```python
from build123d import *

# Parameters (mm, degrees)
SKETCH1_W           = 100
SKETCH1_H           = 100
BOSS_EXTRUDE1_DEPTH = 1.6
CUT_EXTRUDE1_DEPTH  = 1.6
SKETCH7_R           = 1.5875
CUT_EXTRUDE2_DEPTH  = 1.6
SKETCH8_W           = 32
SKETCH8_H           = 6
BOSS_EXTRUDE2_DEPTH = 5
BOSS_EXTRUDE3_DEPTH = 2
SKETCH12_W          = 20
SKETCH12_H          = 6
BOSS_EXTRUDE5_DEPTH = 2


with BuildPart() as part:
    # Sketch1 → Boss-Extrude1 (new body)
    with BuildSketch(Plane.XY):
        with Locations((15.275668243, 27.330907947)):
            Rectangle(SKETCH1_W, SKETCH1_H)
    extrude(amount=BOSS_EXTRUDE1_DEPTH)

    # Sketch2 → Cut-Extrude1 (cut)
    with BuildSketch(Plane.XY.offset(1.6)):
        Polygon((-34.724331757, 57.330907947), (-14.724331757, 77.330907947), (-34.724331757, 77.330907947), align=None)
        Polygon((-34.724331757, -2.669092053), (-14.724331757, -22.669092053), (-34.724331757, -22.669092053), align=None)
        Polygon((45.275668243, 77.330907947), (65.275668243, 57.330907947), (65.275668243, 77.330907947), align=None)
        Polygon((65.275668243, -2.669092053), (45.275668243, -22.669092053), (65.275668243, -22.669092053), align=None)
    extrude(amount=-CUT_EXTRUDE1_DEPTH, mode=Mode.SUBTRACT)

    # Sketch7 → Cut-Extrude2 (cut)
    with BuildSketch(Plane.XY.offset(1.6)):
        with Locations((-25.724331757, 34.330907947)):
            Circle(SKETCH7_R)
        with Locations((-16.624331757, 64.904907947)):
            Circle(SKETCH7_R)
        with Locations((34.275668243, 69.330907947)):
            Circle(SKETCH7_R)
        with Locations((54.275668243, 29.330907947)):
            Circle(SKETCH7_R)
        with Locations((62.999668243, 19.180907947)):
            Circle(SKETCH7_R)
        with Locations((-4.300331757, -20.219092053)):
            Circle(SKETCH7_R)
        with Locations((4.275668243, -5.669092053)):
            Circle(SKETCH7_R)
    extrude(amount=-CUT_EXTRUDE2_DEPTH, mode=Mode.SUBTRACT)

    # Sketch8 → Boss-Extrude2 (add)
    with BuildSketch(Plane.XY.offset(1.6)):
        with Locations((12.949668243, 27.580907947)):
            Rectangle(SKETCH8_W, SKETCH8_H)
    extrude(amount=BOSS_EXTRUDE2_DEPTH)

    # Sketch10 → Boss-Extrude3 (add)
    with BuildSketch(Plane.XY.offset(1.6)):
        Polygon((-34.724331757, 57.330907947), (-14.724331757, 77.330907947), (-12.603011413, 75.209587604), (-32.603011413, 55.209587604), align=None)
        Polygon((45.275668243, 77.330907947), (65.275668243, 57.330907947), (63.154347899, 55.209587604), (43.154347899, 75.209587604), align=None)
        Polygon((65.275668243, -2.669092053), (45.275668243, -22.669092053), (43.154347899, -20.547771709), (63.154347899, -0.547771709), align=None)
        Polygon((-14.724331757, -22.669092053), (-34.724331757, -2.669092053), (-32.603011413, -0.547771709), (-12.603011413, -20.547771709), align=None)
    extrude(amount=BOSS_EXTRUDE3_DEPTH)

    # Sketch12 → Boss-Extrude5 (add)
    with BuildSketch(Plane.XY.offset(1.6)):
        with Locations((16.275668243, 74.330907947)):
            Rectangle(SKETCH12_W, SKETCH12_H)
    extrude(amount=BOSS_EXTRUDE5_DEPTH)


solid = part.part
```
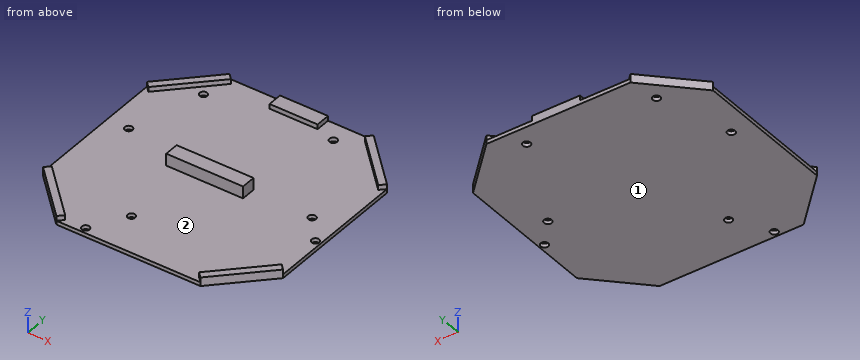
The listing builds one solid part. Answer for the finished solid, in the listing's coordinates (mm). Face numbers are marked on the shaded views. Give positions to 0.01 mm unless a question says otherwise; leave off trailing zeros. Loops run counter-clockwise (first coordinate to the right, second up) from the corner with the lowest first, then second, coordinate; pieces in that order, holes last. Notation, with made-up numbers: (2, 30.25) - (23, 30.25) arc R14 ccw to (23, 43.25) - close; hole circle Ø5 at (49, -11). An arc over 180 degrees is marked (long way). Return JSON: item names as keys, results as strings. Group by question number.
1. Determine the mould class of the marked faces 1 and 2 for opening direction Y: pulls with the +Y half, pulls with the -Y half, needs draft (parallel to the pull), parting line crosses it, or undercut.
2. Find section B-B (x = 22.5). Write down the section's boundary in (y, z), then the cut area to 3 significant figures.
3. Find section A-A (x = 4.5). Write down the section's boundary in (y, z), then the cut area to 3 significant figures.
4. Find section C-C (y = -14.5). Write down the section's boundary in (x, z), then the cut area to 3 significant figures.
5. Find section D-D (x = -17). Write down the section's boundary in (y, z), then the cut area to 3 significant figures.
6. Given pin 1 Ø12 at (x, y) = (28.5, 21.5) entering from +Z; pin 2 Ø3 at (x, y) = (54.28, 29.33) entering from -Z; pin 3 Ø4 at (x, y) = (63, 19.18) entering from +Z; pin 4 Ø1.5 at (x, z) = (8.5, 5) entering from +Y, each flat-ended and moving along its own axis, determine where each tip first touches the part or whether it passes through.
7. Straight lines are drawn through the part: line 1 (Y direction, x = 15, z = 2.5); line 2 (Z direction, x = 4.5, y = 41); line 3 (Y direction, x = 2.5, z = 2.5). For each, find the intervals that lie inside material, in ascending order. Write a range as [from, to].
Verdict:
{
 "1": {"face 1": "needs draft", "face 2": "undercut"},
 "2": {"outline": "(-22.67, 0) - (77.33, 0) - (77.33, 3.6) - (71.33, 3.6) - (71.33, 1.6) - (30.58, 1.6) - (30.58, 6.6) - (24.58, 6.6) - (24.58, 1.6) - (-22.67, 1.6) - close", "area": "202 mm^2"},
 "3": {"outline": "(-22.67, 0) - (-7.24, 0) - (-7.24, 1.6) - (-22.67, 1.6) - close; (-4.1, 0) - (77.33, 0) - (77.33, 1.6) - (30.58, 1.6) - (30.58, 6.6) - (24.58, 6.6) - (24.58, 1.6) - (-4.1, 1.6) - close", "area": "185 mm^2"},
 "4": {"outline": "(-22.89, 0) - (53.44, 0) - (53.44, 3.6) - (49.2, 3.6) - (49.2, 1.6) - (-18.65, 1.6) - (-18.65, 3.6) - (-22.89, 3.6) - close", "area": "139 mm^2"},
 "5": {"outline": "(-20.39, 0) - (63.36, 0) - (63.36, 1.6) - (-16.15, 1.6) - (-16.15, 3.6) - (-20.39, 3.6) - close; (66.45, 0) - (75.06, 0) - (75.06, 3.6) - (70.81, 3.6) - (70.81, 1.6) - (66.45, 1.6) - close", "area": "165 mm^2"},
 "6": {"pin 1": "stops at z = 6.6", "pin 2": "passes through", "pin 3": "stops at z = 1.6", "pin 4": "stops at y = 30.58"},
 "7": {"line 1": "y = [24.58, 30.58], [71.33, 77.33]", "line 2": "z = [0, 1.6]", "line 3": "y = [24.58, 30.58]"}
}
